For this review, use the dimensioned drawing (mm, ordinates from the lowest corner) and the shaded views. A direction names the side the tool comes from. Coordinates: 2 decimals unless noted, no trailing zeros. Loops run counter-clockwise (first coordinate to the right, second up) from the corner with the lowest first, then second, coordinate; pieces in that order, holes last. Notation, with made-up numbers: (21, 69.5) - (36, 69.5) arc R23 cw to (36, 107.5) - close; hole circle Ø11 at (2.5, 7). An arc over 180 degrees is marked (long way). Use one line per item in the form item = value. Start each with the question number.
(1) Tool access review of the marked faces 1 and 2: name each direction out of +Z, -Z, +X, -X, +Y, -Y from which nothing blocks a thin tool from reaching the whole face with its end or side.
(2) For L1, parallel to X at y = 3.5, z = 3.75; L2, parallel to Y at x = 34, z = 0.75, list the stretches that pass through material, from the lowest coordinate up.
(3) Add section B-B (y = 13.5). State the section outline as (x, z) points, plus the area to 3 significant figures.
(4) Add section C-C (y = 8.75). State the section outline as (x, z) points, plus the area to 3 significant figures.
(5) Clearance check with a flat-ended pin moving along its axis: pin 1 Ø1.9 at (y, z) = (7, 4.5) entering from -X. State where the tip first meets the part, or that it passes through.
(6) Add section A-A (z = 0.75). State the section outline as (x, y) points (1 decimal).
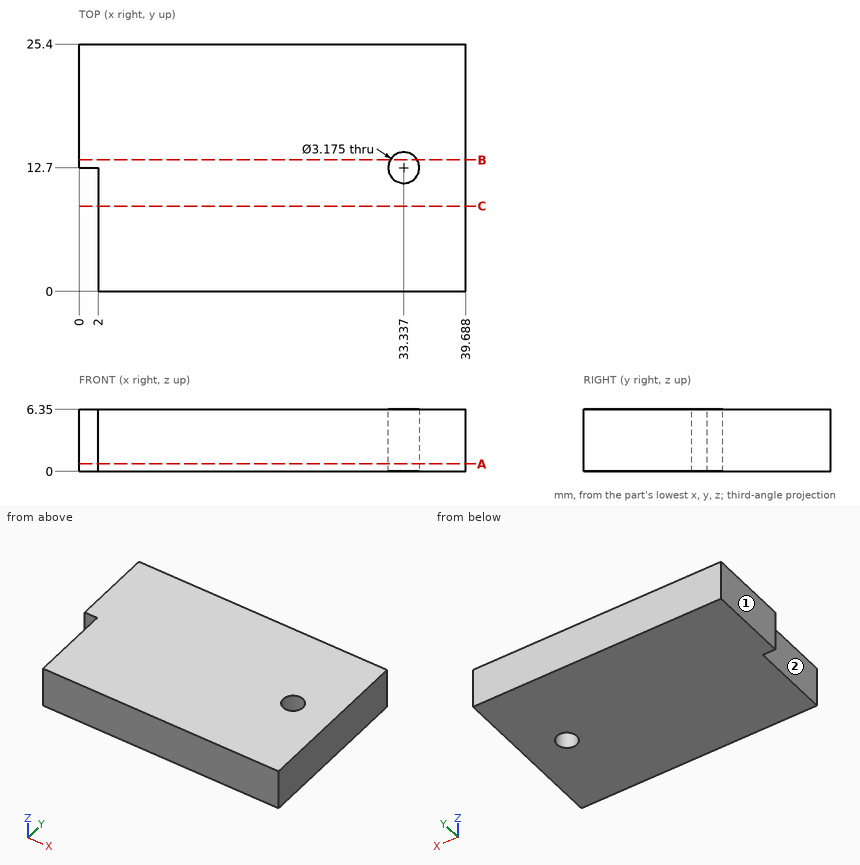
Computed values:
q1.face_1 = +Z, -Z, -X, +Y, -Y
q1.face_2 = +Z, -Z, -X, -Y
q2.L1 = 2 to 39.69
q2.L2 = 0 to 11.26, 14.14 to 25.4
q3.outline = (0, 0) - (31.97, 0) - (31.97, 6.35) - (0, 6.35) - close; (34.71, 0) - (39.69, 0) - (39.69, 6.35) - (34.71, 6.35) - close
q3.area = 235 mm^2
q4.outline = (2, 0) - (39.69, 0) - (39.69, 6.35) - (2, 6.35) - close
q4.area = 239 mm^2
q5.pin_1 = 2
q6.outline = (0, 12.7) - (2, 12.7) - (2, 0) - (39.7, 0) - (39.7, 25.4) - (0, 25.4) - close; hole circle Ø3.2 at (33.3, 12.7)
